Part model, mm, in its own coordinate system. Face numbers are marked on the shaded views. A direction names the side the tool comes from. Round coordinates to 2 decimals unless told otherwise and drop trailing zeros. Write each loop counter-clockwise with the first axis right and the second up, starting at its lowest first coordinate (ties: lowest second). Pieces come first, ordered by that corner, then holes. Notation, with made-up numbers: (50, -3) -> (64, -3) arc R31 ccw to (64, 31) -> close; hole circle Ø3 at (-31, 26). An arc over 180 degrees is marked (long way). Return JSON: item names as keys, results as strings. Group by question number.
```python
from build123d import *

# Parameters (mm, degrees)
SKETCH1_R                                      = 25.4
BOSS_EXTRUDE1_DEPTH                            = 63.5
SKETCH2_R                                      = 14.097
CUT_EXTRUDE1_DEPTH                             = 63.5
SKETCH4_W                                      = 20.32
SKETCH4_H                                      = 43.18
CUT_EXTRUDE3_DEPTH                             = 75.876167103
SKETCH8_R                                      = 14.097
BOSS_EXTRUDE3_DEPTH                            = 10.16
SKETCH10_R                                     = 16.256
BOSS_EXTRUDE4_DEPTH                            = 9.525
SKETCH26_R                                     = 11.7475
BOSS_EXTRUDE8_DEPTH                            = 1.190625
SKETCH11_R                                     = 6.35
BOSS_EXTRUDE5_DEPTH                            = 4.7625
CBORE_FOR_8_SOCKET_HEAD_CAP_SCREW1_D           = 4.4958
CBORE_FOR_8_SOCKET_HEAD_CAP_SCREW1_CBORE_D     = 7.9375
CBORE_FOR_8_SOCKET_HEAD_CAP_SCREW1_CBORE_DEPTH = 22.475825
SKETCH17_W                                     = 3.048
SKETCH17_H                                     = 0.508
CIRPATTERN1_COUNT                              = 2
CIRPATTERN1_ANGLE                              = 90
CHAMFER1_SIZE                                  = 0.508


# Read off the part's stored shape, not the designer's step: 1/4-20 Tapped Hole1, 3/8-24 Tapped Hole1
with BuildPart() as part:
    # Sketch1 → Boss-Extrude1 (new body)
    with BuildSketch(Plane.XY):
        Circle(SKETCH1_R)
    extrude(amount=BOSS_EXTRUDE1_DEPTH)

    # Sketch2 → Cut-Extrude1 (cut)
    with BuildSketch(Plane.XY.offset(63.5)):
        Circle(SKETCH2_R)
    extrude(amount=-CUT_EXTRUDE1_DEPTH, mode=Mode.SUBTRACT)

    # Sketch4 → Cut-Extrude3 (cut, through all)
    with BuildSketch(Plane(origin=(0, 5.08, 0), x_dir=(1, 0, 0), z_dir=(0, 1, 0))):
        with Locations((-15.24, -31.75)):
            Rectangle(SKETCH4_W, SKETCH4_H)
        with Locations((15.24, -31.75)):
            Rectangle(SKETCH4_W, SKETCH4_H)
    cut_extrude3 = extrude(amount=CUT_EXTRUDE3_DEPTH, mode=Mode.SUBTRACT)

    # Mirror1: Cut-Extrude3 across plane
    add(cut_extrude3.mirror(Plane.ZX), mode=Mode.SUBTRACT)

    # Sketch8 → Boss-Extrude3 (add)
    with BuildSketch(Plane.XY.offset(63.5)):
        Circle(SKETCH8_R)
    extrude(amount=-BOSS_EXTRUDE3_DEPTH)

    # Sketch10 → Boss-Extrude4 (add)
    with BuildSketch(Plane.XY.offset(63.5)):
        with Locations(Location((0, 0, 0), (0, 0, 180))):
            Circle(SKETCH10_R)
    extrude(amount=BOSS_EXTRUDE4_DEPTH)

    # Sketch26 → Boss-Extrude8 (add)
    with BuildSketch(Plane.XY.offset(73.025)):
        with Locations(Location((0, 0, 0), (0, 0, 180))):
            Circle(SKETCH26_R)
    extrude(amount=BOSS_EXTRUDE8_DEPTH)

    # Sketch11 → Boss-Extrude5 (add)
    with BuildSketch(Plane.XY.offset(74.215625)):
        with Locations(Location((0, 0, 0), (0, 0, 180))):
            Circle(SKETCH11_R)
    extrude(amount=BOSS_EXTRUDE5_DEPTH)

    # CBORE for #8 Socket Head Cap Screw1 (through all)
    with Locations(Plane.XY.offset(78.978125)):
        with Locations((0, 0)):
            CounterBoreHole(CBORE_FOR_8_SOCKET_HEAD_CAP_SCREW1_D / 2, CBORE_FOR_8_SOCKET_HEAD_CAP_SCREW1_CBORE_D / 2, CBORE_FOR_8_SOCKET_HEAD_CAP_SCREW1_CBORE_DEPTH)

    # Sketch17 → Cut-Revolve5 (revolve, cut)
    with BuildSketch(Plane(origin=(0, 0, 0), x_dir=(0, 0, -1), z_dir=(1, 0, 0)), mode=Mode.PRIVATE) as cut_revolve5_sk:
        with Locations((-58.42, 25.313514496)):
            Rectangle(SKETCH17_W, SKETCH17_H)
        with Locations((-5.08, 25.313514496)):
            Rectangle(SKETCH17_W, SKETCH17_H)
    revolve(cut_revolve5_sk.sketch.rotate(Axis((0, 0, 78.978125), (0, 0, -1)), 90), axis=Axis((0, 0, 78.978125), (0, 0, -1)), mode=Mode.SUBTRACT)

    # 1/4-20 Tapped Hole1 outline → 1/4-20 Tapped Hole1 (revolve, cut)
    with BuildSketch(Plane.YX.offset(-68.2625)):
        Polygon((0, -16.256120693), (3.302120693, -16.256120693), (2.5527, -15.5067), (2.5527, -3.038383775), (0, -3.038383775), align=None)
    f_1_4_20_tapped_hole1 = revolve(axis=Axis((0, 0, 68.2625), (1, 0, 0)), mode=Mode.SUBTRACT)

    # 3/8-24 Tapped Hole1 outline → 3/8-24 Tapped Hole1 (revolve, cut)
    with BuildSketch(Plane.XZ):
        Polygon((3.96875, 56.5023), (4.2164, 56.5023), (4.2164, 77.797025), (5.3975, 78.978125), (3.96875, 78.978125), align=None)
    revolve(axis=Axis((0, 0, 0), (0, 0, 1)), mode=Mode.SUBTRACT)

    # CirPattern1: 1/4-20 Tapped Hole1 ×2 about axis
    cirpattern1_axis = Axis((0, 0, 73.025), (0, 0, -1))
    for i in range(1, CIRPATTERN1_COUNT):
        add(f_1_4_20_tapped_hole1.rotate(cirpattern1_axis, i * CIRPATTERN1_ANGLE / (CIRPATTERN1_COUNT - 1)), mode=Mode.SUBTRACT)

    # Chamfer1
    chamfer1_edges = [part.edges().sort_by_distance(p)[0] for p in [
        (6.35, 0, 78.978125),
    ]]
    chamfer(chamfer1_edges, length=CHAMFER1_SIZE)


solid = part.part
```
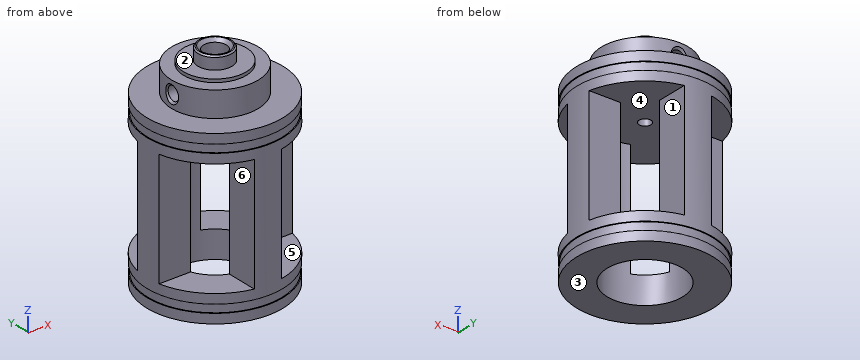
Item 1: Cut at D-D (y = 20). Write the cut outline in (x, z).
Item 2: Wall check: L1, parallel to Z at x = 7, y = 16; L2, parallel to Y at x = 0, z = 39; L3, parallel to X at y = -0.5, z = 45. Give the ranges that are in metal, low to high.
Item 3: Cut at B-B (y = 0). State how many separate pieces and enclosed holes the cut face has, then the cut area to 3 significant figures.
Item 4: Cut at C-C (x = 18.5). Write the cut outline in (y, z).
Item 5: Cut at A-A (z = 40.5). Write the cut outline in (x, y).
Item 6: Two-plate mould, pull along Z, no slides. Class the marked faces 1, 2 and 3: released by +Z, released by -Z, zero draft, split by the parting line, or undercut.
Item 7: Flat gauge pins, fed straight in: P1, Ø16, axis at x = -11, y = 15, coming from the +Z side; P2, Ø9.5, axis at x = 20, z = 25.5, coming from the -Y side; P3, Ø6, axis at y = -19.5, z = 31.5, coming from the -X side; P4, Ø1, axis at x = 15.5, y = 14, coming from the -Z side. Where does each tip first touch, or does it go through?
Item 8: Which spindle directions (+Z, -Z, +X, -X, +Y, -Y) get a long thin tool onto all of the face, cutting with end or side? Do the marked faces 4, 5 and 6. Say none if no direction does.
Checks:
{
 "1": {"outline": "(-15.66, 0) -> (15.66, 0) -> (15.66, 3.56) -> (15.1, 3.56) -> (15.1, 6.6) -> (15.66, 6.6) -> (15.66, 10.16) -> (5.08, 10.16) -> (5.08, 53.34) -> (15.66, 53.34) -> (15.66, 56.9) -> (15.1, 56.9) -> (15.1, 59.94) -> (15.66, 59.94) -> (15.66, 63.5) -> (-15.66, 63.5) -> (-15.66, 59.94) -> (-15.1, 59.94) -> (-15.1, 56.9) -> (-15.66, 56.9) -> (-15.66, 53.34) -> (-5.08, 53.34) -> (-5.08, 10.16) -> (-15.66, 10.16) -> (-15.66, 6.6) -> (-15.1, 6.6) -> (-15.1, 3.56) -> (-15.66, 3.56) -> close"},
 "2": {"L1": "z = 0 to 10.16, 53.34 to 63.5", "L2": "y = -25.4 to -14.1, 14.1 to 25.4", "L3": "x = -25.4 to -14.09, 14.09 to 25.4"},
 "3": {"separate pieces": "3", "enclosed holes": "0", "area": "1,850 mm2"},
 "4": {"outline": "(-17.4, 0) -> (17.4, 0) -> (17.4, 3.56) -> (16.9, 3.56) -> (16.9, 6.6) -> (17.4, 6.6) -> (17.4, 10.16) -> (5.08, 10.16) -> (5.08, 53.34) -> (17.4, 53.34) -> (17.4, 56.9) -> (16.9, 56.9) -> (16.9, 59.94) -> (17.4, 59.94) -> (17.4, 63.5) -> (-17.4, 63.5) -> (-17.4, 59.94) -> (-16.9, 59.94) -> (-16.9, 56.9) -> (-17.4, 56.9) -> (-17.4, 53.34) -> (-5.08, 53.34) -> (-5.08, 10.16) -> (-17.4, 10.16) -> (-17.4, 6.6) -> (-16.9, 6.6) -> (-16.9, 3.56) -> (-17.4, 3.56) -> close"},
 "5": {"outline": "(-24.89, -5.08) -> (-13.15, -5.08) arc R14.1 cw to (-13.15, 5.08) -> (-24.89, 5.08) arc R25.4 ccw to start; (-5.08, -24.89) arc R25.4 ccw to (5.08, -24.89) -> (5.08, -13.15) arc R14.1 cw to (-5.08, -13.15) -> close; (-5.08, 13.15) arc R14.1 cw to (5.08, 13.15) -> (5.08, 24.89) arc R25.4 ccw to (-5.08, 24.89) -> close; (13.15, -5.08) -> (24.89, -5.08) arc R25.4 ccw to (24.89, 5.08) -> (13.15, 5.08) arc R14.1 cw to start"},
 "6": {"face 1": "undercut", "face 2": "released by +Z", "face 3": "released by -Z"},
 "7": {"P1": "stops at z = 74.22", "P2": "stops at y = -5.08", "P3": "stops at x = -5.08", "P4": "stops at z = 0"},
 "8": {"face 4": "none", "face 5": "+X, -Y", "face 6": "-X, +Y, -Y"}
}
